Verification items for the finished model (mm, model axes). Face numbers are marked on the shaded views. A direction names the side the tool comes from. Round coordinates to 2 decimals unless told otherwise and drop trailing zeros. Write each loop counter-clockwise with the first axis right and the second up, starting at its lowest first coordinate (ties: lowest second). Pieces come first, ordered by that corner, then holes.
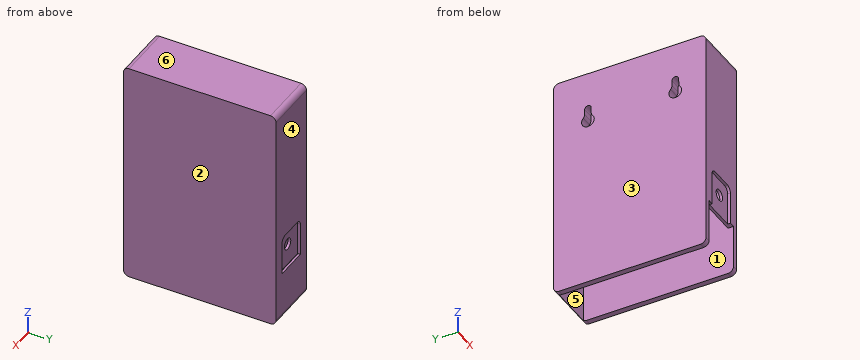
Autodesk Inventor part; units mm, degrees
ref_plane "YZ Plane" through (0, 0, 0) normal (1, 0, 0) x (0, 1, 0)
ref_plane "XZ Plane" through (0, 0, 0) normal (0, 1, 0) x (-1, 0, 0)
ref_plane "XY Plane" through (0, 0, 0) normal (0, 0, 1) x (1, 0, 0)
sketch "Sketch1" plane through (0, 0, 0) normal (1, 0, 0) x (0, 1, 0)
  line L0 (56.5592, 58.2464) -> (-32.0868, 58.2464)
  line L1 (-32.0868, 58.2464) -> (-32.0868, -73.0716)
  line L2 (-32.0868, -73.0716) -> (56.5592, -73.0716)
  line L3 (56.5592, -73.0716) -> (56.5592, 58.2464)
  point P0 (0, 0)
  dimension "d0" = 131.318
  dimension "d1" = 88.646
extrude "Extrusion1" add sketch "Sketch1" along normal blind 31.75
sketch "Sketch2" plane through (0, -32.0868, -73.0716) normal (0, -1, 0) x (1, 0, 0)
  line L0 (31.75, 131.318) -> (31.75, 0)
  line L1 (0, 131.318) -> (0, 0)
  line L2 (28.575, 28.575) -> (3.175, 28.575)
  line L3 (3.175, 28.575) -> (3.175, 0)
  line L4 (3.175, 0) -> (28.575, 0)
  line L5 (28.575, 0) -> (28.575, 28.575)
  point P0 (0, 73.0716)
  point P1 (31.75, 28.575)
  dimension "d7" = 3.175
  dimension "d8" = 3.175
  dimension "d9" = 28.575
extrude "Extrusion2" cut sketch "Sketch2" against normal blind 87.3125
sketch "Sketch3" plane through (28.575, -32.0868, -44.4966) normal (0, 0, -1) x (-1, 0, 0)
  line L0 (0, 0) -> (0, 87.3125)
  line L1 (25.4, 0) -> (25.4, 87.3125)
  line L2 (0, 3.175) -> (25.4, 3.175)
  line L3 (25.4, 3.175) -> (25.4, 84.1375)
  line L4 (25.4, 84.1375) -> (0, 84.1375)
  line L5 (0, 84.1375) -> (0, 3.175)
  line L6 (0, 87.3125) -> (25.4, 87.3125)
  line L7 (25.4, 0) -> (0, 0)
  point P0 (28.575, 32.0868)
  point P1 (12.7, 84.1375)
  point P2 (12.7, 3.175)
  point P3 (0, 84.1375)
  point P4 (25.4, 3.175)
  dimension "d10" = 3.175
  dimension "d11" = 3.175
extrude "Extrusion3" cut sketch "Sketch3" against normal blind 47.625 contours L0 L4 L1 L2
sketch "Sketch4" plane through (0, -32.0868, -73.0716) normal (0, -1, 0) x (1, 0, 0)
  line L0 (3.175, 28.575) -> (28.575, 28.575)
  line L1 (25.4, 28.575) -> (6.35, 28.575)
  line L2 (6.35, 28.575) -> (6.35, 50.8)
  line L3 (6.35, 50.8) -> (25.4, 50.8)
  line L4 (25.4, 50.8) -> (25.4, 28.575)
  line L5 (31.75, 131.318) -> (31.75, 0)
  circle A0 centre (16.7802, 41.275) radius 3.302
  point P0 (0, 73.0716)
  point P1 (15.875, 50.8)
  point P2 (15.875, 28.575)
  point P3 (25.4, 39.6875)
  point P4 (6.35, 28.575)
  dimension "d14" = 22.225
  dimension "d15" = 19.05
  dimension "d16" = 6.35
  dimension "d17" = 6.604
  dimension "d18" = 12.7
extrude "Extrusion4" cut sketch "Sketch4" against normal blind 1.5875
sketch "Sketch6" plane through (0, -30.4993, -73.0716) normal (0, -1, 0) x (1, 0, 0)
  circle A0 centre (16.7802, 41.275) radius 3.302
  circle A1 centre (16.7802, 41.275) radius 3.302
  point P0 (0, 73.0716)
extrude "Extrusion5" cut sketch "Sketch6" along normal mid plane 3.175
ref_plane "Work Plane2" through (0, 12.2362, -73.0716) normal (0, -1, 0) x (1, 0, 0)
mirror "Mirror1" about plane through (0, 12.2362, -73.0716) normal (0, -1, 0) of "Extrusion4"
mirror "Mirror2" about plane through (0, 12.2362, -73.0716) normal (0, -1, 0) of "Extrusion5"
fillet "Fillet1" radius 3.175 3 edges at (30.1625, -32.0868, -73.0716) (1.5875, -32.0868, -73.0716) (15.875, 56.5592, -73.0716)
fillet "Fillet2" radius 3.175 2 edges at (15.875, -32.0868, 58.2464) (15.875, 56.5592, 58.2464)
fillet "Fillet3" radius 3.175 4 edges at (6.35, -31.293, -22.2716) (25.4, -31.293, -22.2716) (25.4, 55.7655, -22.2716) (6.35, 55.7655, -22.2716)
sketch "Sketch8" plane through (0, 0, 0) normal (-1, 0, 0) x (0, 0, 1)
  line L0 (-69.8966, 56.5592) -> (55.0714, 56.5592)
  line L1 (-73.0716, -28.9118) -> (-73.0716, 53.3842)
  arc A0 (31.0026, -11.5151) -> (30.8894, -17.07) centre (28.5284, -14.2433) ccw
  arc A1 (36.1718, -16.1481) -> (36.1484, -12.3383) centre (36.1484, -14.2433) ccw
  line L2 (36.1484, -12.3383) -> (33.1356, -12.3383)
  line L3 (36.1718, -16.1481) -> (32.75, -16.3367)
  arc A2 (31.0026, -11.5151) -> (33.1356, -12.3383) centre (33.1356, -9.1633) ccw
  arc A3 (32.75, -16.3367) -> (30.8894, -17.07) centre (32.9247, -19.5068) ccw
  line L4 (55.0714, -32.0868) -> (-69.8966, -32.0868)
  arc A4 (31.0026, 39.2849) -> (31.0026, 33.8286) centre (28.5284, 36.5567) ccw
  arc A5 (36.1484, 34.6517) -> (36.1484, 38.4617) centre (36.1484, 36.5567) ccw
  line L5 (36.1484, 38.4617) -> (33.1356, 38.4617)
  line L6 (36.1484, 34.6517) -> (33.1356, 34.6517)
  arc A6 (31.0026, 39.2849) -> (33.1356, 38.4617) centre (33.1356, 41.6367) ccw
  arc A7 (33.1356, 34.6517) -> (31.0026, 33.8286) centre (33.1356, 31.4767) ccw
  point P0 (0, 0)
  point P1 (31.6805, -12.3383)
  point P2 (31.5103, -16.405)
  point P3 (31.8314, 36.8525)
  point P4 (31.2779, 32.7727)
  point P5 (31.6805, 38.4617)
  point P6 (31.6805, 34.6517)
  dimension "d57" = 3.81
  dimension "d58" = 7.366
  dimension "d59" = 3.175
  dimension "d60" = 101.6
  dimension "d61" = 109.22
  dimension "d63" = 0
  dimension "d77" = 101.6
  dimension "d78" = 109.22
  dimension "d79" = 50.8
  dimension "d80" = 20.0025
  dimension "d81" = 3.81
  dimension "d82" = 7.366
  dimension "d83" = 3.175
extrude "Extrusion7" cut sketch "Sketch8" against normal blind 6.4008
properties part number "cDAQ_Chassis_LowPolyPlaceholder"
Q1. Release check for a two-part mould opening along X. For the marked faces 1, 2, 3 and 4 record: released by +X, released by -X, zero draft, split by the parting line, or undercut.
Recorded:
face 1: undercut
face 2: released by +X
face 3: released by -X
face 4: zero draft
Q2. Sectioned sample at C-C (y = -14.5). Enter the section's corners in (x, z) (3 decimals).
Recorded:
outline: (0, -73.072) - (3.175, -73.072) - (3.175, 3.128) - (28.575, 3.128) - (28.575, -73.072) - (31.75, -73.072) - (31.75, 58.246) - (0, 58.246) - (0, 38.036) - (6.401, 38.036) - (6.401, 24.854) - (0, 24.854) - close
Q3. Tool access check on the marked faces 5 and 6. Record the directions out of +Z, -Z, +X, -X, +Y, -Y that give a thin tool (end or side, any length) a straight path to the whole face; none if there is none.
Recorded:
face 5: -Z, -Y
face 6: +Z, +X, -X, +Y, -Y
Q4. Sectioned sample at A-A (z = -38.5). Enter the section's corners in (x, y) (3 decimals).
Recorded:
outline: (0, -32.087) - (6.35, -32.087) - (6.35, -30.499) - (25.4, -30.499) - (25.4, -32.087) - (31.75, -32.087) - (31.75, 56.559) - (25.4, 56.559) - (25.4, 54.972) - (6.35, 54.972) - (6.35, 56.559) - (0, 56.559) - close; hole (3.175, -28.912) - (28.575, -28.912) - (28.575, 52.051) - (3.175, 52.051) - close
Q5. Material ranges on line 1 along Y through (x, z) = (13, -14.5); line 2 along X through (y, z) = (-28, -37.5) (3 decimals); line 3 along Y through (x, z) = (9.5, -27), recorded low to high.
Recorded:
line 1: y = -32.09 to -28.91, 52.05 to 56.56
line 2: x = 0 to 3.175, 28.575 to 31.75
line 3: y = -30.5 to -28.91, 52.05 to 54.97
Q6. Sectioned sample at B-B (y = 43.5). Enter the section's corners in (x, z) (3 decimals), plus the area to 3 significant figures.
Recorded:
outline: (0, -73.072) - (3.175, -73.072) - (3.175, 3.128) - (28.575, 3.128) - (28.575, -73.072) - (31.75, -73.072) - (31.75, 58.246) - (0, 58.246) - close
area: 2,230 mm2
Q7. Depth check by flat-ended pin: P1, Ø5.5, axis at x = 16.78, z = -31.8, coming from the -Y side; P2, Ø3.5, axis at x = 15, z = -33, coming from the +Y side; P3, Ø3.5, axis at x = 13, y = -31, coming from the -Z side. Enter the tip coordinate at first touch or a pass-through.
Recorded:
P1: stops at y = 52.05
P2: stops at y = 54.97
P3: stops at z = -44.5
